Design review of the part shown in the three views and the two pictorial views. Dimensions are in mm from the part's minimum x, y and z. A direction names the side the tool comes from. Coordinates: 2 decimals unless noted, no trailing zeros. Write each loop counter-clockwise with the first axis right and the second up, starting at its lowest first coordinate (ties: lowest second). Pieces come first, ordered by that corner, then holes. Notation, with made-up numbers: M 1,39 L 10,39 A21 ccw 10,76 Z; hole C 60.5,-12.5 d10. An arc over 180 degrees is marked long. Answer as a JSON object with one key per item and string values.
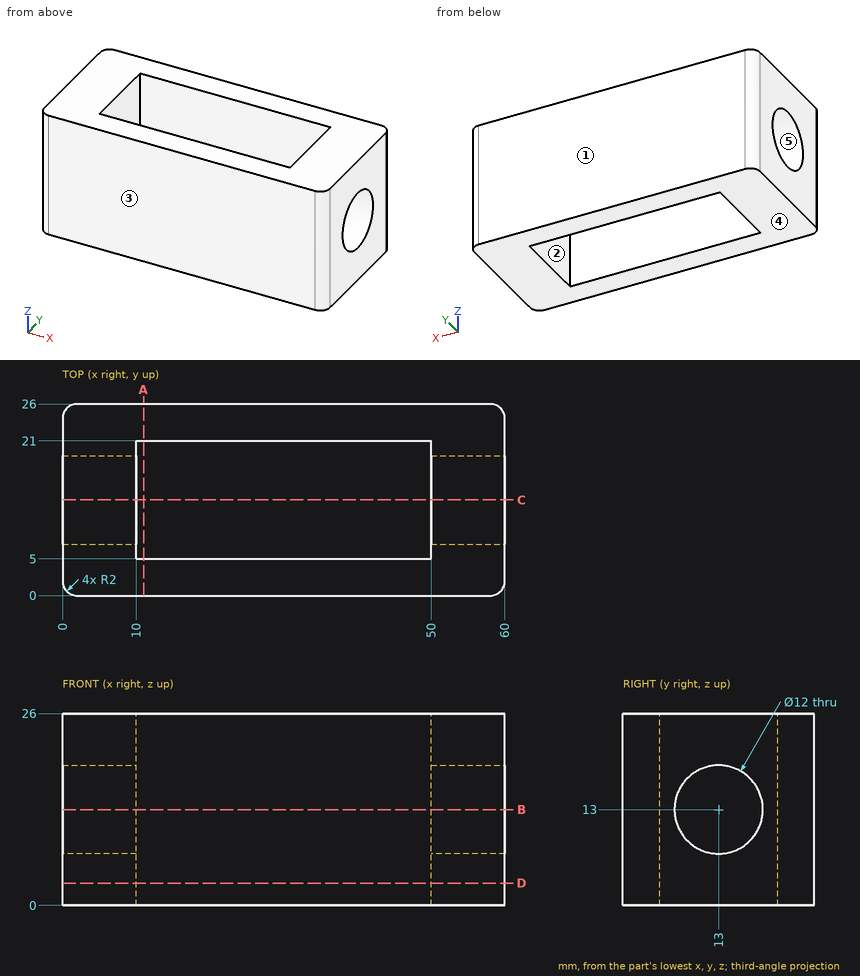
(1) Add section D-D on z = 3. Give the boundary of the cut face in (x, y).
Results list:
{"outline": "M 0,2 A2 ccw 2,0 L 58,0 A2 ccw 60,2 L 60,24 A2 ccw 58,26 L 2,26 A2 ccw 0,24 Z; hole M 10,5 L 50,5 L 50,21 L 10,21 Z"}
(2) Draft analysis for pull direction Z (two halves, no side actions). For the marked faces 3, 4 and 5, state which applies: released by +Z, released by -Z, zero draft, split by the parting line, or undercut.
Results list:
{"face 3": "zero draft", "face 4": "released by -Z", "face 5": "undercut"}
(3) For the marked faces 1 and 2, list the 3-axis set-ups (+Z, -Z, +X, -X, +Y, -Y) from which the entire face can be reached by the end or side of a thin tool; tool diameter is ignored.
Results list:
{"face 1": "+Z, -Z, +X, -X, +Y", "face 2": "+Z, -Z"}
(4) Wall thickness on line 1 along Y through (x, z) = (56.25, 13); line 2 along X through (y, z) = (11.5, 1.25); line 3 along Y through (x, z) = (23, 6.5): over which ranges is each line inside the solid? List them lowest first. Write a range as from..to.
Results list:
{"line 1": "0..7, 19..26", "line 2": "0..10, 50..60", "line 3": "0..5, 21..26"}
(5) Add section B-B on z = 13. Give the boundary of the cut face in (x, y).
Results list:
{"outline": "M 0,2 A2 ccw 2,0 L 58,0 A2 ccw 60,2 L 60,7 L 50,7 L 50,5 L 10,5 L 10,7 L 0,7 Z; M 0,19 L 10,19 L 10,21 L 50,21 L 50,19 L 60,19 L 60,24 A2 ccw 58,26 L 2,26 A2 ccw 0,24 Z"}
(6) Add section C-C on y = 13. Give the boundary of the cut face in (x, z), and give its area (3 significant figures).
Results list:
{"outline": "M 0,0 L 10,0 L 10,7 L 0,7 Z; M 0,19 L 10,19 L 10,26 L 0,26 Z; M 50,0 L 60,0 L 60,7 L 50,7 Z; M 50,19 L 60,19 L 60,26 L 50,26 Z", "area": "280 mm²"}
(7) Add section A-A on x = 11. Give the boundary of the cut face in (y, z).
Results list:
{"outline": "M 0,0 L 5,0 L 5,26 L 0,26 Z; M 21,0 L 26,0 L 26,26 L 21,26 Z"}
